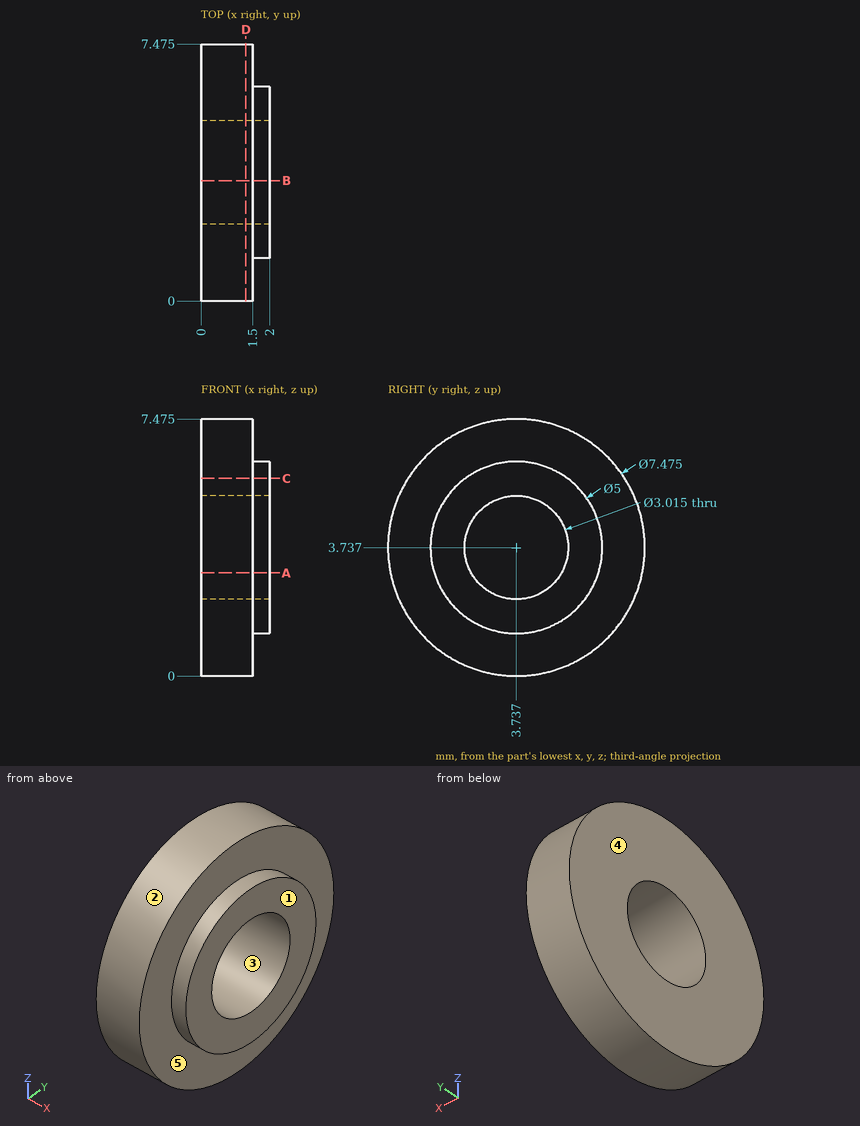
For this review, use the dimensioned drawing (mm, ordinates from the lowest corner) and the shaded views. A direction names the side the tool comes from. Give positions to 0.01 mm unless a question says otherwise; leave off trailing zeros. Order: outer loops, then holes, each group sorted by start corner. A loop starts at its lowest first (then second) coordinate and runs counter-clockwise, first axis right, second up.
1) Take a section at D-D (x = 1.3). Give the boundary of the cut face in (y, z) (1 decimal).
2) For the marked faces 4 and 5, list the 3-axis set-ups (+Z, -Z, +X, -X, +Y, -Y) from which the entire face can be reached by the end or side of a thin tool; tool diameter is ignored.
3) Take a section at A-A (z = 3). Give the boundary of the cut face in (x, y).
4) Take a section at C-C (z = 5.75). Give the boundary of the cut face in (x, y) (1 decimal), then the cut area to 3 significant figures.
5) Insertion check: pin 1 (1 mm diameter, centred on x = 1.5, y = 5.5, fed in from +Z) (1 decimal). The pin has a flat end and moves straight along its axis. Give the tip position at first contact, or say it passes through.
6) Take a section at B-B (y = 3.5). Give the boundary of the cut face in (x, z).
7) The part is to be moulded in two halves that separate along Y. For the marked faces 1, 2 and 3, say which applies: released by +Y, released by -Y, zero draft, split by the parting line, or undercut.
8) Wall thickness on line 1 (X direction, y = 1, z = 2.5); line 2 (Y direction, x = 0.65, z = 4.5) (1 decimal); line 3 (Z direction, x = 1.4, y = 3) (1 decimal): over which ranges is each line inside the solid? List them lowest first.
Derived:
1. outline: circle Ø7.5 at (3.7, 3.7); hole circle Ø3 at (3.7, 3.7)
2. face 4: +Z, -Z, -X, +Y, -Y
2. face 5: +X
3. outline: (0, 0.07) - (1.5, 0.07) - (1.5, 1.35) - (2, 1.35) - (2, 2.42) - (0, 2.42) - close; (0, 5.05) - (2, 5.05) - (2, 6.13) - (1.5, 6.13) - (1.5, 7.4) - (0, 7.4) - close
4. outline: (0, 0.6) - (1.5, 0.6) - (1.5, 2.3) - (2, 2.3) - (2, 5.2) - (1.5, 5.2) - (1.5, 6.9) - (0, 6.9) - close
4. area: 10.9 mm2
5. pin 1: stops at z = 7.3
6. outline: (0, 0.01) - (1.5, 0.01) - (1.5, 1.25) - (2, 1.25) - (2, 2.25) - (0, 2.25) - close; (0, 5.23) - (2, 5.23) - (2, 6.23) - (1.5, 6.23) - (1.5, 7.47) - (0, 7.47) - close
7. face 1: zero draft
7. face 2: split by the parting line
7. face 3: undercut
8. line 1: x = 0 to 1.5
8. line 2: y = 0.1 to 2.4, 5 to 7.4
8. line 3: z = 0.1 to 2.4, 5.1 to 7.4
